Geometry: see drawing. Coordinates: mm, zero at the bounding-box minimum. Give positions to 0.01 mm unless a question says otherwise; leave off trailing zeros. Write each loop counter-clockwise with the first axis right and the second up, starting at its lowest first coordinate (ties: lowest second). Pieces come first, ordered by that corner, then holes. Notation, with made-up numbers: M 41.5,23.25 L 59.5,23.25 A3 ccw 59.5,27.25 Z; hole C 16.5,-25.5 d10. An arc over 180 degrees is marked long. Use a Markdown table: item, result. Add a question column.
(1) Cut plane C-C (x = 85.5). Output: boundary loops of the cut face in (y, z), plus the area to 3 significant figures.
(2) Draft query along Y for the marked faces 1, 2, 3 and 4. Return one class per face: released by +Y, released by -Y, zero draft, split by the parting line, or undercut.
(3) Cut plane B-B (x = 6). Output: boundary loops of the cut face in (y, z).
(4) Cut plane A-A (z = 10). Output: boundary loops of the cut face in (x, y).
(5) Pin query (flat end, axial travel): pin 1 Ø15 at (y, z) = (17.5, 18.5) entering from -X. Return the tip coordinate at first contact, or that it passes through.
(6) Cut plane D-D (z = 28.5). Output: boundary loops of the cut face in (x, y), plus the area to 3 significant figures.
(7) Material intervals for L1, parallel to X at y = 0.75, z = 50; L2, parallel to Z at x = 34, y = 53; L3, parallel to Y at x = 40.5, z = 55.5, sorted ascending.
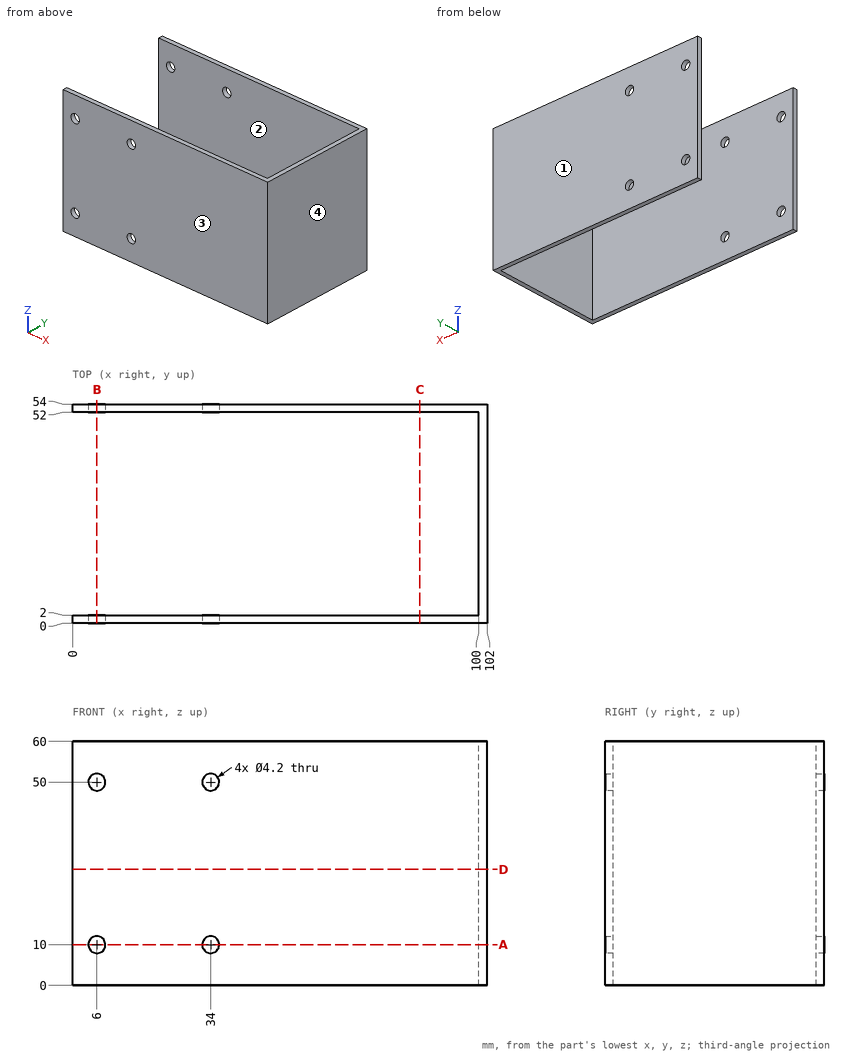
Answer list:
| question | item | result |
|---|---|---|
| 1 | outline | M 0,0 L 2,0 L 2,60 L 0,60 Z; M 52,0 L 54,0 L 54,60 L 52,60 Z |
| 1 | area | 240 mm² |
| 2 | face 1 | released by +Y |
| 2 | face 2 | undercut |
| 2 | face 3 | released by -Y |
| 2 | face 4 | zero draft |
| 3 | outline | M 0,0 L 2,0 L 2,7.9 L 0,7.9 Z; M 0,12.1 L 2,12.1 L 2,47.9 L 0,47.9 Z; M 0,52.1 L 2,52.1 L 2,60 L 0,60 Z; M 52,0 L 54,0 L 54,7.9 L 52,7.9 Z; M 52,12.1 L 54,12.1 L 54,47.9 L 52,47.9 Z; M 52,52.1 L 54,52.1 L 54,60 L 52,60 Z |
| 4 | outline | M 0,0 L 3.9,0 L 3.9,2 L 0,2 Z; M 0,52 L 3.9,52 L 3.9,54 L 0,54 Z; M 8.1,0 L 31.9,0 L 31.9,2 L 8.1,2 Z; M 8.1,52 L 31.9,52 L 31.9,54 L 8.1,54 Z; M 36.1,0 L 102,0 L 102,54 L 36.1,54 L 36.1,52 L 100,52 L 100,2 L 36.1,2 Z |
| 5 | pin 1 | x = 100 |
| 6 | outline | M 0,0 L 102,0 L 102,54 L 0,54 L 0,52 L 100,52 L 100,2 L 0,2 Z |
| 6 | area | 508 mm² |
| 7 | L1 | 0 to 3.9, 8.1 to 31.9, 36.1 to 102 |
| 7 | L2 | 0 to 7.9, 12.1 to 47.9, 52.1 to 60 |
| 7 | L3 | 0 to 2, 52 to 54 |
